Part print with two shaded views. Sizes in mm from the minimum x, y, z corner. Round coordinates to 2 decimals unless told otherwise and drop trailing zeros. One line per question, with ' | ' between items. Start each with the question number.
1) Wall check: probe 1 along Y at (x, z) = (1.35, 13.25); probe 2 along Y at (x, z) = (2.2, 9.5); probe 3 along Z at (x, y) = (1.9, 13.75). Give the ranges that are in metal, low to high. Write a range as [from, to].
2) Drop a flat-ended pin along its axis: pin 1 Ø1.5 at (x, y) = (2, 8.5) entering from +Z. Give the stop position or say it passes through.
3) Mould opens along Z. For the marked faces 1, 2 and 3 say: pulls with the +Z half, pulls with the -Z half, needs draft (parallel to the pull), parting line crosses it, or undercut.
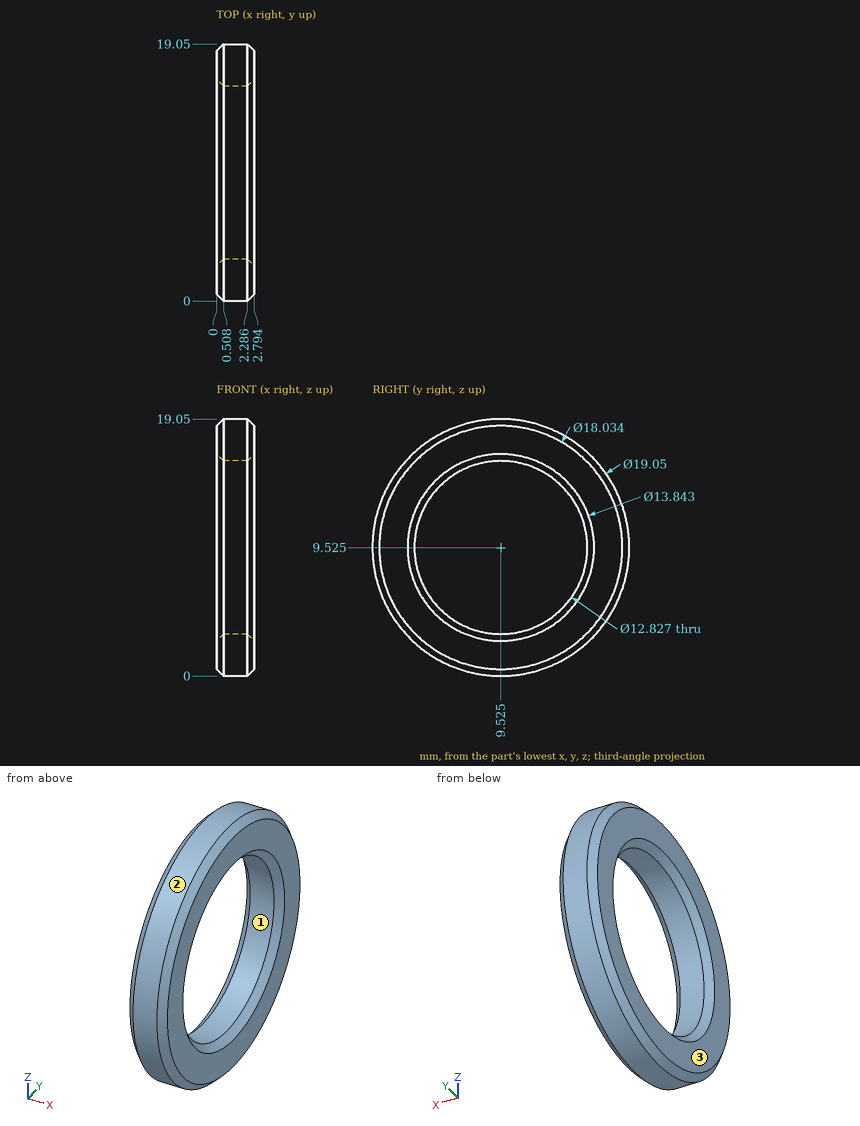
Answer key:
1) probe 1: y = [0.76, 4.3], [14.75, 18.29] | probe 2: y = [0, 3.11], [15.94, 19.05] | probe 3: z = [0.99, 4.7], [14.35, 18.06]
2) pin 1: stops at z = 19.05
3) face 1: undercut | face 2: parting line crosses it | face 3: needs draft
